```python
from build123d import *

# Parameters (mm, degrees)
SKETCH1_R           = 22.5
BOSS_EXTRUDE1_DEPTH = 25
SKETCH2_R           = 12.5
CUT_EXTRUDE1_DEPTH  = 10
FILLET1_R           = 5
SKETCH3_R           = 1.5
CUT_EXTRUDE2_DEPTH  = 41.466035196


with BuildPart() as part:
    # Sketch1 → Boss-Extrude1 (new body)
    with BuildSketch(Plane(origin=(0, 0, 0), x_dir=(0, 0, -1), z_dir=(1, 0, 0))):
        Circle(SKETCH1_R)
    extrude(amount=BOSS_EXTRUDE1_DEPTH)

    # Sketch2 → Cut-Extrude1 (cut)
    with BuildSketch(Plane(origin=(25, 0, 0), x_dir=(0, 0, -1), z_dir=(1, 0, 0))):
        Circle(SKETCH2_R)
    extrude(amount=-CUT_EXTRUDE1_DEPTH, mode=Mode.SUBTRACT)

    # Fillet1
    fillet1_edges = [part.edges().sort_by_distance(p)[0] for p in [
        (0, 0, 22.5),
        (25, 0, 22.5),
    ]]
    fillet(fillet1_edges, radius=FILLET1_R)

    # Sketch3 → Cut-Extrude2 (cut, through all)
    with BuildSketch(Plane.ZY):
        Circle(SKETCH3_R)
    extrude(amount=-CUT_EXTRUDE2_DEPTH, mode=Mode.SUBTRACT)


solid = part.part
```
Build history of the part. All positions in model axes, mm. A direction names the side the tool comes from. Coordinates: 2 decimals unless noted, no trailing zeros. Order: outer loops, then holes, each group sorted by start corner. A loop starts at its lowest first (then second) coordinate and runs counter-clockwise, first axis right, second up. Notation, with made-up numbers: M 16.25,12.25 L 22.25,12.25 A32 cw 22.25,39.25 Z; hole C 36.5,-35.5 d8. An arc over 180 degrees is marked long. One line per question, with ' | ' between items. Start each with the question number.
1. Wall check: line 1 along Y through (x, z) = (7.25, 0); line 2 along Y through (x, z) = (17.25, 0); line 3 along X through (y, z) = (6.5, -5). Give the ranges that are in metal, low to high. Write a range as [from, to].
2. Cut at D-D (x = 17.25). Write the cut outline in (y, z), plus the area to 3 significant figures.
3. Mould opens along Z. For faces 3 (the face through (12.395, -19.961, -10.382)), 4 (the face through (7.4, 0.07, -1.5)), 5 (the face through (0, -4, 0)) say: +Z half, -Z half, draft (parallel to the pull), parting line (faces both ways), or undercut.
4. Cut at A-A (y = 0). Write the cut outline in (x, z), plus the area to 3 significant figures.
5. Tool access for faces 1 (the face through (25, -8, -11)), 2 (the face through (15, -3, 0)): list every direction of +Z, -Z, +X, -X, +Y, -Y with a clear straight run to the whole face (end or side of a thin tool).
6. Flat gauge pins, fed straight in: P1, Ø2, axis at x = 13.5, z = -8, coming from the -Y side; P2, Ø1, axis at x = 3.5, z = -14.5, coming from the -Y side; P3, Ø2, axis at x = 22, z = 9, coming from the -Y side. Where does each tip first touch, or does it go through?
7. Cut at C-C (x = 9.5). Write the cut outline in (y, z).
The answers:
1) line 1: y = [-22.5, -1.5], [1.5, 22.5] | line 2: y = [-22.5, -12.5], [12.5, 22.5] | line 3: x = [0, 15]
2) outline: C 0,0 d45; hole C 0,0 d25 | area: 1,100 mm2
3) face 3: parting line | face 4: undercut | face 5: draft
4) outline: M 0,-17.5 A5 ccw 5,-22.5 L 20,-22.5 A5 ccw 25,-17.5 L 25,-12.5 L 15,-12.5 L 15,-1.5 L 0,-1.5 Z; M 0,1.5 L 15,1.5 L 15,12.5 L 25,12.5 L 25,17.5 A5 ccw 20,22.5 L 5,22.5 A5 ccw 0,17.5 Z | area: 809 mm2
5) face 1: +Z, -Z, +X, +Y, -Y | face 2: +X
6) P1: stops at y = -21.38 | P2: stops at y = -17.36 | P3: stops at y = -20.74
7) outline: C 0,0 d45; hole C 0,0 d3
